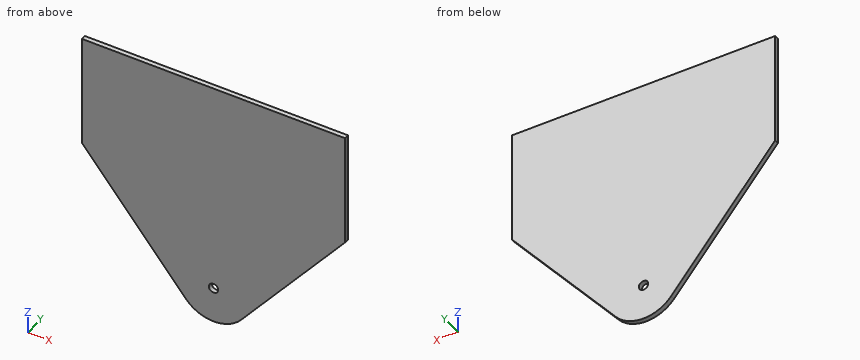
from build123d import *

# Parameters (mm, degrees)
SKETCH1_R           = 3.175
BOSS_EXTRUDE1_DEPTH = 3.175


with BuildPart() as part:
    # Sketch1 → Boss-Extrude1 (new body)
    with BuildSketch(Plane(origin=(0, 0, 0), x_dir=(1, 0, 0), z_dir=(0, 1, 0))):
        with BuildLine():
            Line((-88.9, 0), (88.9, 0))
            Line((88.9, 0), (88.9, 76.2))
            Line((88.9, 76.2), (18.702682169, 161.291999073))
            ThreePointArc((18.702682169, 161.291999073), (0, 170.108527998), (-18.702682169, 161.291999073))
            Line((-18.702682169, 161.291999073), (-88.9, 76.2))
            Line((-88.9, 76.2), (-88.9, 0))
        make_face()
        with Locations(Location((0, 145.863073453, 0), (0, 0, 270))):
            Circle(SKETCH1_R, mode=Mode.SUBTRACT)
    extrude(amount=BOSS_EXTRUDE1_DEPTH)


solid = part.part
Source: CAD feature listing. Evaluate the final solid. Frame: model axes, mm. Round coordinates to 2 decimals unless told otherwise and drop trailing zeros. Loops run counter-clockwise (first coordinate to the right, second up) from the corner with the lowest first, then second, coordinate; pieces in that order, holes last. Notation, with made-up numbers: M -3.5,81 L 27.5,81 A34 ccw 27.5,119 Z; hole C 46.5,21 d3. An arc over 180 degrees is marked long. Return JSON: item names as keys, results as strings. Group by question number.
1. Section query D-D on x = 47.5. Output: boundary loops of the cut face in (y, z) (3 decimals).
2. Section query B-B on y = 1.6. Output: boundary loops of the cut face in (x, z) (3 decimals), and give its area (3 significant figures).
3. Section query A-A on x = 0. Output: boundary loops of the cut face in (y, z) (3 decimals).
4. Section query C-C on z = -125.5. Output: boundary loops of the cut face in (x, y) (3 decimals), and give its area (3 significant figures).
5. Material intervals for line 1 along X through (y, z) = (2.8, -142.5); line 2 along Z through (x, y) = (-36, 0.2); line 3 along X through (y, z) = (0.8, -116), sorted ascending. Write a range as from..to.
Checks:
{
 "1": {"outline": "M 0,-126.384 L 3.175,-126.384 L 3.175,0 L 0,0 Z"},
 "2": {"outline": "M -88.9,-76.2 L -18.703,-161.292 A24.245 ccw 18.703,-161.292 L 88.9,-76.2 L 88.9,0 L -88.9,0 Z; hole C 0,-145.863 d6.35", "area": "22,900 mm²"},
 "3": {"outline": "M 0,-170.109 L 3.175,-170.109 L 3.175,-149.038 L 0,-149.038 Z; M 0,-142.688 L 3.175,-142.688 L 3.175,0 L 0,0 Z"},
 "4": {"outline": "M -48.23,0 L 48.23,0 L 48.23,3.175 L -48.23,3.175 Z", "area": "306 mm²"},
 "5": {"line 1": "x = -34.21..34.21", "line 2": "z = -140.32..0", "line 3": "x = -56.07..56.07"}
}
